The drawing under review shows one solid part. Ordinate dimensions are in mm from its lowest x, y, z. A direction names the side the tool comes from. Coordinates: 2 decimals unless noted, no trailing zeros. Write each loop counter-clockwise with the first axis right and the second up, starting at its lowest first coordinate (ties: lowest second). Pieces come first, ordered by that corner, then holes. Notation, with made-up numbers: (1.25, -33.75) - (21.25, -33.75) arc R26 ccw to (21.25, 4.25) - close; hole circle Ø11 at (-21.5, -16). An arc over 180 degrees is marked (long way). Put each result on its own line as item: value. Start each with the question number.
Item 1: For pin 1 (5 mm diameter, centred on x = 21, z = 9.5, fed in from -Y); pin 2 (10 mm diameter, centred on x = 15.5, y = 44.5, fed in from +Z); pin 3 (5 mm diameter, centred on x = 26, y = 14.5, fed in from +Z); pin 4 (1.5 mm diameter, centred on x = 25, z = 8, fed in from +Y), all flat-tipped, find the tip position at first contact; note any pin that passes through.
Item 2: To check wall thickness, follow L1, parallel to X at y = 47.5, z = 7.25; L2, parallel to Y at x = 10, z = 7.25; L3, parallel to Z at x = 21.5, y = 26. State the ranges of each line that lie inside material, in increasing order. Write a range as [from, to].
Item 3: Consider section D-D on z = 3. Give the boundary of the cut face in (x, y), then the cut area to 3 significant figures.
Item 4: Consider section A-A on z = 7. Give the boundary of the cut face in (x, y), then the cut area to 3 significant figures.
Item 5: Consider section C-C on y = 46. Give the boundary of the cut face in (x, z).
Item 6: Machinability: for the marked faces 1, 2, 3 and 4, which of the approach directions +Z, -Z, +X, -X, +Y, -Y give a long, thin tool a straight path to every point of the face, cutting with its end or side? Answer none if there is none.
Item 7: Consider section B-B on x = 13. Give the boundary of the cut face in (y, z), then the cut area to 3 significant figures.
Item 8: Mouldability with a two-part tool opening along X and no side actions: class the marked faces 5, 6 and 7 as pulls with the +X half, pulls with the -X half, needs draft (parallel to the pull), parting line crosses it, or undercut.
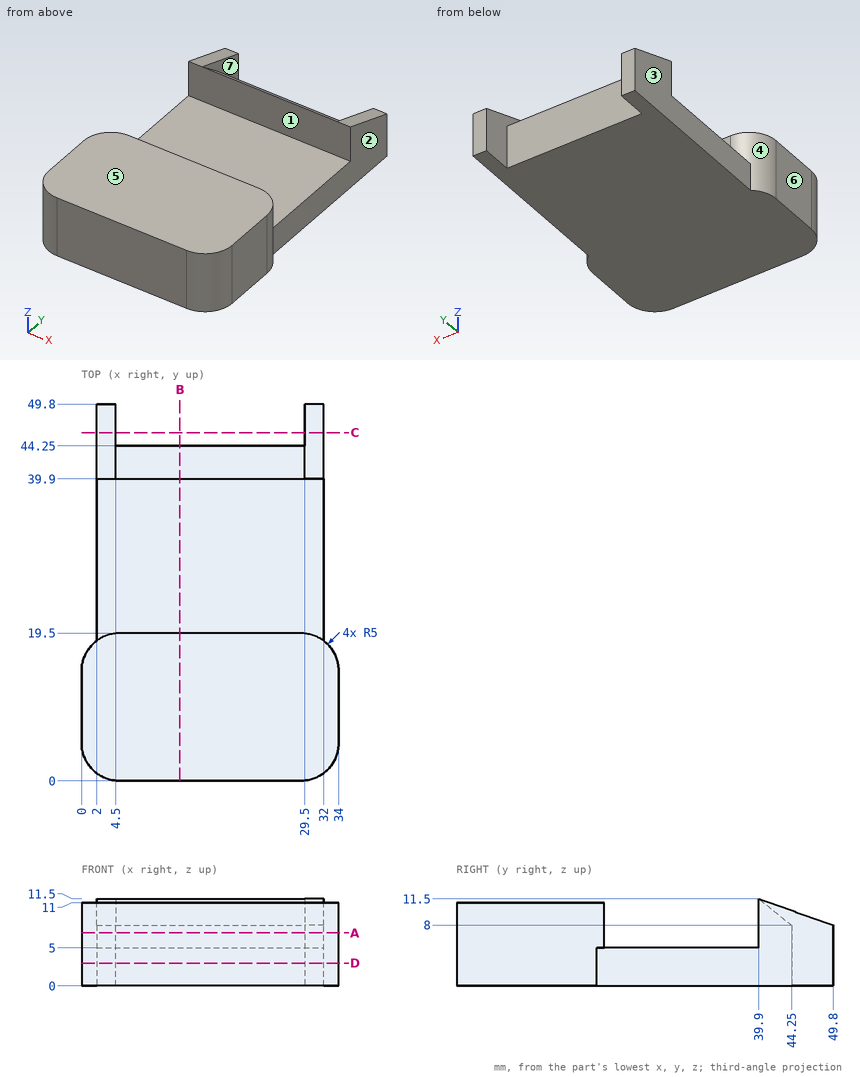
Report:
1. pin 1: y = 0
1. pin 2: z = 11.5
1. pin 3: z = 11
1. pin 4: y = 44.25
2. L1: [2, 4.5], [29.5, 32]
2. L2: [0, 19.5], [39.9, 44.25]
2. L3: [0, 5]
3. outline: (0, 5) arc R5 ccw to (5, 0) - (29, 0) arc R5 ccw to (34, 5) - (34, 14.5) arc R5 ccw to (32, 18.5) - (32, 49.8) - (29.5, 49.8) - (29.5, 44.25) - (4.5, 44.25) - (4.5, 49.8) - (2, 49.8) - (2, 18.5) arc R5 ccw to (0, 14.5) - close
3. area: 1,410 mm²
4. outline: (0, 5) arc R5 ccw to (5, 0) - (29, 0) arc R5 ccw to (34, 5) - (34, 14.5) arc R5 ccw to (29, 19.5) - (5, 19.5) arc R5 ccw to (0, 14.5) - close; (2, 39.9) - (32, 39.9) - (32, 49.8) - (29.5, 49.8) - (29.5, 44.25) - (4.5, 44.25) - (4.5, 49.8) - (2, 49.8) - close
4. area: 800 mm²
5. outline: (2, 0) - (4.5, 0) - (4.5, 9.34) - (2, 9.34) - close; (29.5, 0) - (32, 0) - (32, 9.34) - (29.5, 9.34) - close
6. face 1: +Z, +X, -X
6. face 2: +Z, -Z, +X, +Y
6. face 3: +Z, -Z, -X, +Y
6. face 4: +Z, -X
7. outline: (0, 0) - (44.25, 0) - (44.25, 8) - (39.9, 11.5) - (39.9, 5) - (19.5, 5) - (19.5, 11) - (0, 11) - close
7. area: 359 mm²
8. face 5: needs draft
8. face 6: pulls with the -X half
8. face 7: undercut
